```python
from build123d import *

# Parameters (mm, degrees)
SKETCH_1_W          = 20
SKETCH_1_H          = 20
EXTRUDE_1_DEPTH     = 80
SKETCH_2_R          = 2.1
CUT_EXTRUDE_1_DEPTH = 84.066238629
SKETCH_3_W          = 18
SKETCH_3_H          = 18
CUT_EXTRUDE_2_DEPTH = 82.240384046


with BuildPart() as part:
    # 草图1 → 凸台-拉伸1 (new body)
    with BuildSketch(Plane.XY):
        Rectangle(SKETCH_1_W, SKETCH_1_H)
    extrude(amount=EXTRUDE_1_DEPTH)

    # 草图2 → 切除-拉伸1 (cut, through all)
    with BuildSketch(Plane(origin=(10, 0, 0), x_dir=(0, 0, -1), z_dir=(1, 0, 0))):
        with Locations((-70, 0)):
            Circle(SKETCH_2_R)
        with Locations((-10, 0)):
            Circle(SKETCH_2_R)
        with Locations((-50, 0)):
            Circle(SKETCH_2_R)
        with Locations(Location((-30, 0, 0), (0, 0, 180))):
            Circle(SKETCH_2_R)
    extrude(amount=-CUT_EXTRUDE_1_DEPTH, mode=Mode.SUBTRACT)

    # 草图3 → 切除-拉伸2 (cut, through all)
    with BuildSketch(Plane(origin=(0, 0, 0), x_dir=(-1, 0, 0), z_dir=(0, 0, -1))):
        Rectangle(SKETCH_3_W, SKETCH_3_H)
    extrude(amount=-CUT_EXTRUDE_2_DEPTH, mode=Mode.SUBTRACT)


solid = part.part
```
Input: part model. Units: mm. Frame: model coordinates. A direction names the side the tool comes from. Round coordinates to 2 decimals unless told otherwise and drop trailing zeros. Loops run counter-clockwise (first coordinate to the right, second up) from the corner with the lowest first, then second, coordinate; pieces in that order, holes last. Notation, with made-up numbers: (26, -31) -> (80, -31) arc R25 ccw to (80, -5) -> close; hole circle Ø6 at (49, -17.75). An arc over 180 degrees is marked (long way). One line per item, written item: value.
(1) Section A-A (x = 6.5). Return the cut outline in (y, z).
Geometry check:
outline: (-10, 0) -> (-9, 0) -> (-9, 80) -> (-10, 80) -> close; (9, 0) -> (10, 0) -> (10, 80) -> (9, 80) -> close
(2) Section C-C (z = 16.5). Return the cut outline in (x, y), plus the area to 3 significant figures.
Geometry check:
outline: (-10, -10) -> (10, -10) -> (10, 10) -> (-10, 10) -> close; hole (-9, -9) -> (9, -9) -> (9, 9) -> (-9, 9) -> close
area: 76.0 mm2
(3) Section D-D (z = 30). Return the cut outline in (x, y).
Geometry check:
outline: (-10, -10) -> (10, -10) -> (10, -2.1) -> (9, -2.1) -> (9, -9) -> (-9, -9) -> (-9, -2.1) -> (-10, -2.1) -> close; (-10, 2.1) -> (-9, 2.1) -> (-9, 9) -> (9, 9) -> (9, 2.1) -> (10, 2.1) -> (10, 10) -> (-10, 10) -> close
(4) Material intervals for line 1 (X direction, y = 5.25, z = 17); line 2 (Y direction, x = -9.45, z = 50), sorted ascending. Write a range as [from, to].
Geometry check:
line 1: [-10, -9], [9, 10]
line 2: [-10, -2.1], [2.1, 10]
(5) Mould query, pull axis Y, two halves, no side actions, for faces 3 (the face through (9, 0, 39)), 4 (the face through (0, 10, 39)), 5 (the face through (-0.8, -9.6, 80)), 6 (the face through (0, -10, 39)). Classes: pulls with the +Y half, pulls with the -Y half, needs draft (parallel to the pull), parting line crosses it, or undercut.
Geometry check:
face 3: undercut
face 4: pulls with the +Y half
face 5: needs draft
face 6: pulls with the -Y half
(6) Pin query (flat end, axial travel): pin 1 (6 mm diameter, centred on x = 5, y = 0, fed in from -Z). Return the tip coordinate at first contact, or that it passes through.
Geometry check:
pin 1: through
(7) Set-up query: faces 1 (the face through (0, -9, 39)), 2 (the face through (9.51, 0.09, 72.1)). Return all of +Z, -Z, +X, -X, +Y, -Y with unobstructed straight access to the full face (end or side cutting, diameter ignored); none if empty.
Geometry check:
face 1: +Z, -Z
face 2: +X, -X
